```python
from build123d import *

# Parameters (mm, degrees)
BOSS_EXTRUDE1_DEPTH  = 5.588
SKETCH2_W            = 25.4
SKETCH2_H            = 5.588
CUT_EXTRUDE1_DEPTH   = 103.543043372
M3_CLEARANCE_HOLE1_D = 3.4
M3_CLEARANCE_HOLE2_D = 3.4


with BuildPart() as part:
    # Sketch1 → Boss-Extrude1 (new body)
    with BuildSketch(Plane(origin=(0, 0, 0), x_dir=(1, 0, 0), z_dir=(0, 1, 0))):
        Polygon((19.05, 31.75), (19.05, 50.8), (-19.05, 50.8), (-19.05, 31.75), (-88.9, 31.75), (-88.9, -31.75), (-19.05, -31.75), (-19.05, -50.8), (19.05, -50.8), (19.05, -31.75), (88.9, -31.75), (88.9, 31.75), align=None)
    extrude(amount=BOSS_EXTRUDE1_DEPTH)

    # Sketch2 → Cut-Extrude1 (cut, through all)
    with BuildSketch(Plane(origin=(0, 5.588, 0), x_dir=(1, 0, 0), z_dir=(0, 1, 0))):
        with Locations((0, 44.196)):
            Rectangle(SKETCH2_W, SKETCH2_H)
        with Locations((0, -44.196)):
            Rectangle(SKETCH2_W, SKETCH2_H)
    extrude(amount=-CUT_EXTRUDE1_DEPTH, mode=Mode.SUBTRACT)

    # M3 Clearance Hole1 (through all)
    with Locations(Plane(origin=(0, 5.588, 0), x_dir=(1, 0, 0), z_dir=(0, 1, 0))):
        with Locations((-14.1986, 24.1681), (68.4276, 24.1681), (68.4276, -24.1681), (-6.7056, -24.1681)):
            Hole(M3_CLEARANCE_HOLE1_D / 2)

    # M3 Clearance Hole2 (through all)
    with Locations(Plane(origin=(0, 5.588, 0), x_dir=(1, 0, 0), z_dir=(0, 1, 0))):
        with Locations((-24.765, 12.827), (-82.4865, 12.827)):
            Hole(M3_CLEARANCE_HOLE2_D / 2)


solid = part.part
```
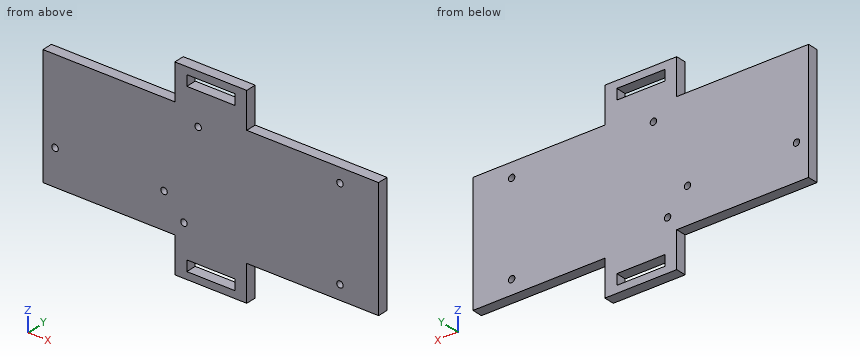
Input: part model. Units: mm. Frame: model coordinates. Give positions to 0.01 mm unless a question says otherwise; leave off trailing zeros. Order: outer loops, then holes, each group sorted by start corner. A loop starts at its lowest first (then second) coordinate and runs counter-clockwise, first axis right, second up.
1. Pin query (flat end, axial travel): pin 1 Ø1.7 at (x, y) = (-45.5, 2) entering from +Z; pin 2 Ø3 at (x, z) = (68.43, -24.17) entering from +Y; pin 3 Ø3 at (y, z) = (3.5, -44) entering from -X. Return the tip coordinate at first contact, or that it passes through.
Computed:
pin 1: stops at z = 31.75
pin 2: passes through
pin 3: stops at x = -19.05
2. Line query: probe 1 along Z at (x, y) = (-11, 3.6); probe 2 along X at (y, z) = (2.6, 44); probe 3 along Z at (x, y) = (20, 0.5). Output: solid intervals per line, ascending.
Computed:
probe 1: z = -50.8 to -46.99, -41.4 to 41.4, 46.99 to 50.8
probe 2: x = -19.05 to -12.7, 12.7 to 19.05
probe 3: z = -31.75 to 31.75
3. Cut plane B-B (y = 1.35). State how many separate pieces and enclosed holes the cut face has, and give its area (3 significant figures).
Computed:
separate pieces: 1
enclosed holes: 8
area: 12,400 mm2
4. Cut plane A-A (x = -10.5). Return loops of the section in (y, z), and give its area (3 significant figures).
Computed:
outline: (0, -50.8) - (5.59, -50.8) - (5.59, -46.99) - (0, -46.99) - close; (0, -41.4) - (5.59, -41.4) - (5.59, 41.4) - (0, 41.4) - close; (0, 46.99) - (5.59, 46.99) - (5.59, 50.8) - (0, 50.8) - close
area: 505 mm2
5. Cut plane C-C (x = 35). Return loops of the section in (y, z).
Computed:
outline: (0, -31.75) - (5.59, -31.75) - (5.59, 31.75) - (0, 31.75) - close
